Here's how the part is built. I have some questions about the finished solid (model axes, mm). A direction names the side the tool comes from. Round coordinates to 2 decimals unless told otherwise and drop trailing zeros. Use a Markdown table: item, result. Add a question column.
(1) Thinking about a two-plate mould opening in X: for faces 3 (the face through (-0.29, 11.72, 6.5)), 4 (the face through (-1, 17, 10)), 5 (the face through (0, 0, 5)), 6 (the face through (-49, -23, 5)), which applies, pulls with the +X half, pulls with the -X half, needs draft (parallel to the pull), parting line crosses it, or undercut?
(2) I'm going to push flat-ended pins straight in: P1, Ø3, axis at x = -7, y = 8, coming from the +Z side; P2, Ø8, axis at x = -7, y = 2, coming from the +Z side. Where does each tip first touch, or does it pass through?
(3) If I drill on probe 1 along X at (y, z) = (3.5, 9.5); probe 2 along X at (y, z) = (1, 9); probe 3 along Y at (x, z) = (-19.5, 8), over which ranges is the centre line in solid material (lowest first)?
(4) On a 3-axis mill with a long thin cutter (end or side, diameter ignored), from which of +Z, -Z, +X, -X, +Y, -Y can I reach the whole of each face in a straight line? I mean faces 1 (the face through (-24.61, -0.11, 6.5)), 2 (the face through (-1, -25, 5)). Say none if no direction works.
from build123d import *

# Parameters (mm, degrees)
F0_W     = 100
F0_H     = 50
F1_DEPTH = 10
F2_R     = 5
F3_W     = 52.0799309015
F3_H     = 26.2977816164
F4_DEPTH = 5
F5_R     = 5
F6_R     = 4.99999


# Not quite as in the source:
# - a fillet or chamfer is up to 0.001 mm smaller than in the source, because OpenCascade refuses the exact size


with BuildPart() as f1:
    # F0 (on Top) → F1 (new body)
    with BuildSketch(Plane.XY):
        Rectangle(F0_W, F0_H)
    extrude(amount=F1_DEPTH)

    # F2
    f2_edges = [f1.edges().sort_by_distance(p)[0] for p in [
        (-50, -25, 5),
        (-50, 25, 5),
        (50, -25, 5),
        (50, 25, 5),
    ]]
    fillet(f2_edges, radius=F2_R)

    # F3 (on face) → F4 (cut)
    with BuildSketch(Plane.XY.offset(10)):
        Rectangle(F3_W, F3_H)
    extrude(amount=-F4_DEPTH, mode=Mode.SUBTRACT)

    # F5
    f5_edges = [f1.edges().sort_by_distance(p)[0] for p in [
        (-26.039965, 13.148891, 7.5),
        (26.039965, 13.148891, 7.5),
        (26.039965, -13.148891, 7.5),
        (-26.039965, -13.148891, 7.5),
    ]]
    fillet(f5_edges, radius=F5_R)

    # F6 (radius 5 in the source; OpenCascade refuses exactly that, so slightly less here)
    f6_edges = [f1.edges().sort_by_distance(p)[0] for p in [
        (0, -13.148891, 5),
        (-24.575499, -11.684425, 5),
        (24.575499, -11.684425, 5),
        (-26.039965, 0, 5),
        (26.039965, 0, 5),
        (-24.575499, 11.684425, 5),
        (24.575499, 11.684425, 5),
        (0, 13.148891, 5),
    ]]
    fillet(f6_edges, radius=F6_R)


solid = f1.part
Taken from the geometry:
| question | item | result |
|---|---|---|
| 1 | face 3 | undercut |
| 1 | face 4 | needs draft |
| 1 | face 5 | undercut |
| 1 | face 6 | pulls with the -X half |
| 2 | P1 | stops at z = 5.19 |
| 2 | P2 | stops at z = 5 |
| 3 | probe 1 | x = -50 to -26.01, 26.01 to 50 |
| 3 | probe 2 | x = -50 to -25.94, 25.94 to 50 |
| 3 | probe 3 | y = -25 to -12.73, 12.73 to 25 |
| 4 | face 1 | +Z |
| 4 | face 2 | +Z, -Z, +X, -X, -Y |
